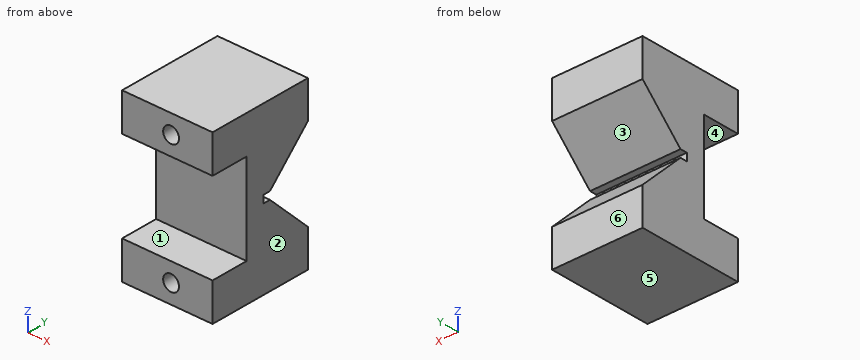
from build123d import *

# Parameters (mm, degrees)
BOSS_EXTRUDE1_DEPTH   = 24
M5_TAPPED_HOLE1_D     = 4.2
M5_TAPPED_HOLE1_DEPTH = 12
M5_TAPPED_HOLE1_TIP   = 1.2618073


with BuildPart() as part:
    # Sketch1 → Boss-Extrude1 (new body)
    with BuildSketch(Plane(origin=(0, 0, 0), x_dir=(0, 0, -1), z_dir=(1, 0, 0))):
        Polygon((12, 10), (-12, 10), (-12, 0), (-22, 0), (-22, 28), (-12.142135624, 28), (-1, 16.857864376), (-1, 15), (1, 15), (1, 16.857864376), (12.142135624, 28), (22, 28), (22, 0), (12, 0), align=None)
    extrude(amount=BOSS_EXTRUDE1_DEPTH)

    # M5 Tapped Hole1
    with Locations(Plane(origin=(0, 0, 0), x_dir=(-1, 0, 0), z_dir=(0, -1, 0))):
        with Locations((-13, 17), (-13, -17)):
            Hole(M5_TAPPED_HOLE1_D / 2, depth=M5_TAPPED_HOLE1_DEPTH)
            with Locations((0, 0, -(M5_TAPPED_HOLE1_DEPTH + M5_TAPPED_HOLE1_TIP / 2))):  # 118° drill point
                Cone(0, M5_TAPPED_HOLE1_D / 2, M5_TAPPED_HOLE1_TIP, mode=Mode.SUBTRACT)


solid = part.part
Part model, mm, in its own coordinate system. Face numbers are marked on the shaded views. A direction names the side the tool comes from. Coordinates: 2 decimals unless noted, no trailing zeros. Loops run counter-clockwise (first coordinate to the right, second up) from the corner with the lowest first, then second, coordinate; pieces in that order, holes last. Notation, with made-up numbers: M 65,-15 L 72,-15 A34 cw 72,24 Z; hole C -39,36 d3. An arc over 180 degrees is marked long. Use a Markdown table: item, result. Add a question column.
Q1. Cut at B-B (x = 5). Write the cut outline in (y, z).
Q2. Cut at C-C (y = 22.25). Write the cut outline in (x, z).
Q3. Pin check, flat tips, straight feed: P1, Ø2, axis at y = 23, z = 3.5, coming from the +X side; P2, Ø1.6, axis at x = 10, z = 0, coming from the +Y side; P3, Ø2.5, axis at x = 13, z = 17, coming from the -Y side; P4, Ø7, axis at x = 9.5, z = -3.5, coming from the -Y side. Stop position of each tip, or through.
Q4. Cut at A-A (y = 7.5). Write the cut outline in (x, z).
Q5. Which spindle directions (+Z, -Z, +X, -X, +Y, -Y) get a long thin tool onto all of the face, cutting with end or side? Do the marked faces 1, 2 and 3. Say none if no direction does.
Q6. Mould opens along Z. For the marked faces 4, 5 and 6 say: +Z half, -Z half, draft (parallel to the pull), parting line (faces both ways), or undercut.
Q7. Probe L1, parallel to Z at x = 13, y = 6; L2, parallel to Z at x = 21.25, y = 4.75; L3, parallel to X at y = 3.75, z = -17. List the from-to ranges inside material, lowest first.
Q8. Cut at D-D (z = 11). Write the cut outline in (x, y).
Worked out:
| question | item | result |
|---|---|---|
| 1 | outline | M 0,-22 L 28,-22 L 28,-12.14 L 16.86,-1 L 15,-1 L 15,1 L 16.86,1 L 28,12.14 L 28,22 L 0,22 L 0,12 L 10,12 L 10,-12 L 0,-12 Z |
| 2 | outline | M 0,-22 L 24,-22 L 24,-6.39 L 0,-6.39 Z; M 0,6.39 L 24,6.39 L 24,22 L 0,22 Z |
| 3 | P1 | passes through |
| 3 | P2 | stops at y = 15 |
| 3 | P3 | stops at y = 12.51 |
| 3 | P4 | stops at y = 10 |
| 4 | outline | M 0,-22 L 24,-22 L 24,-12 L 0,-12 Z; M 0,12 L 24,12 L 24,22 L 0,22 Z; hole C 13,-17 d4.2; hole C 13,17 d4.2 |
| 5 | face 1 | +X, -X, -Y |
| 5 | face 2 | +Z, -Z, +X, +Y, -Y |
| 5 | face 3 | +X, -X, +Y |
| 6 | face 4 | undercut |
| 6 | face 5 | -Z half |
| 6 | face 6 | draft |
| 7 | L1 | z = -22 to -19.1, -14.9 to -12, 12 to 14.9, 19.1 to 22 |
| 7 | L2 | z = -22 to -12, 12 to 22 |
| 7 | L3 | x = 0 to 10.9, 15.1 to 24 |
| 8 | outline | M 0,10 L 24,10 L 24,26.86 L 0,26.86 Z |
